Geometry: final body of the model. Coordinates: model frame, mm. A direction names the side the tool comes from. Give positions to 0.01 mm unless a question says otherwise; leave off trailing zeros. Order: outer loops, then holes, each group sorted by start corner. A loop starts at its lowest first (then second) coordinate and runs counter-clockwise, first axis right, second up. Notation, with made-up numbers: (50.25, 20) - (102.25, 20) arc R20 cw to (102.25, 48) - close; hole circle Ø4 at (-3.75, 75). An arc over 180 degrees is marked (long way). One line per item, written item: value.
Solid Edge part; units mm, degrees
sketch "Sketch1" plane through (0, 0, 0) normal (0, 0, 1) x (1, 0, 0)
  circle A0 centre (0, 0) radius 111
extrude "Protrusion1" add sketch "Sketch1" along normal blind 6
sketch "Sketch2" plane through (0, 0, 6) normal (0, 0, 1) x (1, 0, 0)
  circle A0 centre (0, 0) radius 101
extrude "Cutout1" cut sketch "Sketch2" against normal through all
sketch "Sketch3" plane through (0, 0, 6) normal (0, 0, 1) x (1, 0, 0)
  line L0 (-5, 103) -> (5, 103)
  line L1 (5, 103) -> (5, 109)
  line L2 (5, 109) -> (-5, 109)
  line L3 (-5, 109) -> (-5, 103)
  dimension "D1" = 5
  dimension "D2" = 5
extrude "Cutout2" cut sketch "Sketch3" against normal through all
pattern_circular "Pattern1" count 4 over 360 about axis through (0, 0, 6) along (0, 0, -1) of "Cutout2"
properties material "Wood, Mahogany"
1) Set-up query: faces 4 (the face through (98.1, 25.2, 0)), 5 (the face through (109, 0, 3)). Return all of +Z, -Z, +X, -X, +Y, -Y with unobstructed straight access to the full face (end or side cutting, diameter ignored); none if empty.
Answers below:
face 4: -Z, +X, -X, +Y, -Y
face 5: +Z, -Z
2) Section B-B, the plane y = 0. Return loops of the section in (x, z), then the cut area to 3 significant figures.
Answers below:
outline: (-111, 0) - (-109, 0) - (-109, 6) - (-111, 6) - close; (-103, 0) - (-101, 0) - (-101, 6) - (-103, 6) - close; (101, 0) - (103, 0) - (103, 6) - (101, 6) - close; (109, 0) - (111, 0) - (111, 6) - (109, 6) - close
area: 48.0 mm^2
3) First-contact query: pin 1 (1.8 mm diameter, centred on y = 1, z = 2, fed in from +X); pin 2 (3 mm diameter, centred on y = 88.5, z = 4, fed in from -X); pin 3 (1 mm diameter, centred on x = 55, z = 2, fed in from -Y); pin 4 (2 mm diameter, centred on y = 32, z = 1, fed in from +X). Flat tips, straight axial feed; report the tip coordinate or a pass-through.
Answers below:
pin 1: x = 111
pin 2: x = -68.93
pin 3: y = -96.7
pin 4: x = 106.58
4) Section A-A, the plane z = 0.9. Return loops of the section in (x, y).
Answers below:
outline: circle Ø222 at (0, 0); hole (-109, -5) - (-103, -5) - (-103, 5) - (-109, 5) - close; hole circle Ø202 at (0, 0); hole (-5, -109) - (5, -109) - (5, -103) - (-5, -103) - close; hole (-5, 103) - (5, 103) - (5, 109) - (-5, 109) - close; hole (103, -5) - (109, -5) - (109, 5) - (103, 5) - close
5) Mould query, pull axis X, two halves, no side actions, for faces 1 (the face through (105.874, -33.341, 2.958)), 2 (the face through (98.1, 25.2, 6)), 3 (the face through (5, -106, 3)). Classes: released by +X, released by -X, zero draft, split by the parting line, or undercut.
Answers below:
face 1: split by the parting line
face 2: zero draft
face 3: undercut
6) Material intervals for line 1 along Y through (x, z) = (0, 4); line 2 along X through (y, z) = (81.5, 4.05); line 3 along X through (y, z) = (44, 3.5), sorted ascending.
Answers below:
line 1: -111 to -109, -103 to -101, 101 to 103, 109 to 111
line 2: -75.36 to -59.66, 59.66 to 75.36
line 3: -101.91 to -90.91, 90.91 to 101.91
7) Section D-D, the plane x = -90. Return loops of the section in (y, z), then the cut area to 3 significant figures.
Answers below:
outline: (-64.97, 0) - (-45.84, 0) - (-45.84, 6) - (-64.97, 6) - close; (45.84, 0) - (64.97, 0) - (64.97, 6) - (45.84, 6) - close
area: 230 mm^2
